Geometry: final body of the model. Coordinates: model frame, mm. A direction names the side the tool comes from. Give positions to 0.01 mm unless a question says otherwise; leave off trailing zeros. Write each loop counter-clockwise with the first axis right and the second up, starting at its lowest first coordinate (ties: lowest second). Pieces come first, ordered by that corner, then holes. Notation, with made-up numbers: (-9.5, 14) - (35.5, 14) arc R26 cw to (35.5, 51) - close; hole circle Ø6 at (-24, 28.25). An arc over 180 degrees is marked (long way). Return JSON: item names as keys, results as strings.
Autodesk Inventor part; units mm, degrees
ref_plane "YZ Plane" through (0, 0, 0) normal (1, 0, 0) x (0, 1, 0)
ref_plane "XZ Plane" through (0, 0, 0) normal (0, 1, 0) x (-1, 0, 0)
ref_plane "XY Plane" through (0, 0, 0) normal (0, 0, 1) x (1, 0, 0)
sketch "Sketch1" plane through (0, 0, 0) normal (0, 1, 0) x (-1, 0, 0)
  line L0 (0, 0) -> (-29.0466, 0)
  line L1 (0, 58.5031) -> (-5.7395, 64.2426)
  line L2 (6.2813, 43.0294) -> (-10.3357, 59.6464)
  line L3 (-10.3357, 59.6464) -> (-1.1433, 68.8388)
  line L4 (-1.1433, 68.8388) -> (15.4737, 52.2218)
  line L5 (15.4737, 52.2218) -> (6.2813, 43.0294)
  line L6 (6.2813, 43.0294) -> (-1.1433, 68.8388) construction
  line L7 (-10.3357, 59.6464) -> (15.4737, 52.2218) construction
  line L8 (7.802, 36.0648) -> (-17.3003, 61.1671)
  line L9 (-17.3003, 61.1671) -> (-2.664, 75.8034)
  line L10 (-2.664, 75.8034) -> (22.4383, 50.7011)
  line L11 (22.4383, 50.7011) -> (7.802, 36.0648)
  line L12 (7.802, 36.0648) -> (-2.664, 75.8034) construction
  line L13 (-17.3003, 61.1671) -> (22.4383, 50.7011) construction
  line L14 (7.802, 36.0648) -> (7.802, -0.7306)
  line L15 (22.4383, 50.7011) -> (22.4383, -0.4008)
  line L16 (6.2813, -43.0294) -> (-10.3357, -59.6464)
  line L17 (-10.3357, -59.6464) -> (-1.1433, -68.8388)
  line L18 (-1.1433, -68.8388) -> (15.4737, -52.2218)
  line L19 (15.4737, -52.2218) -> (6.2813, -43.0294)
  line L20 (-10.3357, -59.6464) -> (15.4737, -52.2218) construction
  line L21 (7.802, -36.0648) -> (-17.3003, -61.1671)
  line L22 (-17.3003, -61.1671) -> (-2.664, -75.8034)
  line L23 (-2.664, -75.8034) -> (22.4383, -50.7011)
  line L24 (22.4383, -50.7011) -> (7.802, -36.0648)
  line L25 (7.802, -36.0648) -> (-2.664, -75.8034) construction
  line L26 (7.802, -36.0648) -> (7.802, -0.7306)
  line L27 (22.4383, -50.7011) -> (22.4383, -0.4008)
  point P0 (2.569, 55.9341)
  point P1 (-1.4969, 60)
  dimension "d0" = 45
  dimension "d1" = 6
  dimension "d2" = 23.5
  dimension "d3" = 13
  dimension "d4" = 60
  dimension "d6" = 6
extrude "Extrusion1" add sketch "Sketch1" along normal blind 6
sketch "Sketch3" plane through (0, 0, 0) normal (0, -1, 0) x (1, 0, 0)
  line L0 (-9.3663, 0) -> (-22.4383, 0)
  line L1 (-22.4383, -50.7011) -> (-22.4383, 50.7011)
  circle A0 centre (-15.2967, -35) radius 3.75
  circle A1 centre (-15.2967, 0) radius 3.75
  circle A2 centre (-15.2967, -17.5) radius 3.75
  circle A3 centre (-15.2967, 35) radius 3.75
  line L2 (-19.0467, -35) -> (-17.1717, -31.7524)
  line L3 (-17.1717, -31.7524) -> (-13.4217, -31.7524)
  line L4 (-13.4217, -31.7524) -> (-11.5467, -35)
  line L5 (-11.5467, -35) -> (-13.4217, -38.2476)
  line L6 (-13.4217, -38.2476) -> (-17.1717, -38.2476)
  line L7 (-17.1717, -38.2476) -> (-19.0467, -35)
  line L8 (-19.0467, -17.5) -> (-17.1717, -14.2524)
  line L9 (-17.1717, -14.2524) -> (-13.4217, -14.2524)
  line L10 (-13.4217, -14.2524) -> (-11.5467, -17.5)
  line L11 (-11.5467, -17.5) -> (-13.4217, -20.7476)
  line L12 (-13.4217, -20.7476) -> (-17.1717, -20.7476)
  line L13 (-17.1717, -20.7476) -> (-19.0467, -17.5)
  line L14 (-19.0467, 0) -> (-17.1717, 3.2476)
  line L15 (-17.1717, 3.2476) -> (-13.4217, 3.2476)
  line L16 (-13.4217, 3.2476) -> (-11.5467, 0)
  line L17 (-11.5467, 0) -> (-13.4217, -3.2476)
  line L18 (-13.4217, -3.2476) -> (-17.1717, -3.2476)
  line L19 (-17.1717, -3.2476) -> (-19.0467, 0)
  line L20 (-19.0467, 35) -> (-17.1717, 38.2476)
  line L21 (-17.1717, 38.2476) -> (-13.4217, 38.2476)
  line L22 (-13.4217, 38.2476) -> (-11.5467, 35)
  line L23 (-11.5467, 35) -> (-13.4217, 31.7524)
  line L24 (-13.4217, 31.7524) -> (-17.1717, 31.7524)
  line L25 (-17.1717, 31.7524) -> (-19.0467, 35)
  circle A4 centre (-15.2967, 17.5) radius 3.75
  line L26 (-19.0467, 17.5) -> (-17.1717, 20.7476)
  line L27 (-17.1717, 20.7476) -> (-13.4217, 20.7476)
  line L28 (-13.4217, 20.7476) -> (-11.5467, 17.5)
  line L29 (-11.5467, 17.5) -> (-13.4217, 14.2524)
  line L30 (-13.4217, 14.2524) -> (-17.1717, 14.2524)
  line L31 (-17.1717, 14.2524) -> (-19.0467, 17.5)
  point P0 (0, 0)
  dimension "d15" = 7.5
  dimension "d16" = 7.5
  dimension "d17" = 7.5
  dimension "d19" = 7.5
  dimension "d20" = 7.5
extrude "Extrusion3" cut sketch "Sketch3" against normal blind 6 contours L17 L18 L19 L0 | L0 L14 L15 L16 | L5 L6 L7 L2 L3 L4 | L11 L12 L13 L8 L9 L10 | L23 L24 L25 L20 L21 L22 | L29 L30 L31 L26 L27 L28
sketch "Sketch5" plane through (0, 6, 0) normal (0, 1, 0) x (1, 0, 0)
  line L0 (-17.1717, -3.2476) -> (-19.0467, 0)
  line L1 (-19.0467, 0) -> (-17.1717, 3.2476)
  line L2 (-17.1717, 3.2476) -> (-13.4217, 3.2476)
  line L3 (-13.4217, 3.2476) -> (-11.5467, 0)
  line L4 (-11.5467, 0) -> (-13.4217, -3.2476)
  line L5 (-13.4217, -3.2476) -> (-17.1717, -3.2476)
  line L6 (-13.4217, 20.7476) -> (-11.5467, 17.5)
  line L7 (-11.5467, 17.5) -> (-13.4217, 14.2524)
  line L8 (-13.4217, 14.2524) -> (-17.1717, 14.2524)
  line L9 (-17.1717, 14.2524) -> (-19.0467, 17.5)
  line L10 (-19.0467, 17.5) -> (-17.1717, 20.7476)
  line L11 (-17.1717, 20.7476) -> (-13.4217, 20.7476)
  line L12 (-13.4217, -31.7524) -> (-11.5467, -35)
  line L13 (-11.5467, -35) -> (-13.4217, -38.2476)
  line L14 (-13.4217, -38.2476) -> (-17.1717, -38.2476)
  line L15 (-17.1717, -38.2476) -> (-19.0467, -35)
  line L16 (-19.0467, -35) -> (-17.1717, -31.7524)
  line L17 (-17.1717, -31.7524) -> (-13.4217, -31.7524)
  line L18 (-13.4217, 38.2476) -> (-11.5467, 35)
  line L19 (-11.5467, 35) -> (-13.4217, 31.7524)
  line L20 (-13.4217, 31.7524) -> (-17.1717, 31.7524)
  line L21 (-17.1717, 31.7524) -> (-19.0467, 35)
  line L22 (-19.0467, 35) -> (-17.1717, 38.2476)
  line L23 (-17.1717, 38.2476) -> (-13.4217, 38.2476)
  line L24 (-13.4217, -14.2524) -> (-11.5467, -17.5)
  line L25 (-11.5467, -17.5) -> (-13.4217, -20.7476)
  line L26 (-13.4217, -20.7476) -> (-17.1717, -20.7476)
  line L27 (-17.1717, -20.7476) -> (-19.0467, -17.5)
  line L28 (-19.0467, -17.5) -> (-17.1717, -14.2524)
  line L29 (-17.1717, -14.2524) -> (-13.4217, -14.2524)
  line L30 (-7.802, -36.0648) -> (-7.802, 36.0648)
  line L31 (-7.802, 36.0648) -> (17.3003, 61.1671)
  line L32 (17.3003, 61.1671) -> (2.664, 75.8034)
  line L33 (2.664, 75.8034) -> (-22.4383, 50.7011)
  line L34 (-22.4383, 50.7011) -> (-22.4383, -50.7011)
  line L35 (-22.4383, -50.7011) -> (2.664, -75.8034)
  line L36 (2.664, -75.8034) -> (17.3003, -61.1671)
  line L37 (17.3003, -61.1671) -> (-7.802, -36.0648)
  line L38 (1.1433, 68.8388) -> (10.3357, 59.6464)
  line L39 (10.3357, 59.6464) -> (-6.2813, 43.0294)
  line L40 (-6.2813, 43.0294) -> (-15.4737, 52.2218)
  line L41 (-15.4737, 52.2218) -> (1.1433, 68.8388)
  line L42 (1.1433, -68.8388) -> (-15.4737, -52.2218)
  line L43 (-15.4737, -52.2218) -> (-6.2813, -43.0294)
  line L44 (-6.2813, -43.0294) -> (10.3357, -59.6464)
  line L45 (10.3357, -59.6464) -> (1.1433, -68.8388)
  line L46 (-13.4217, -31.7524) -> (-11.5467, -35)
  line L47 (-11.5467, -35) -> (-7.802, -35)
  line L48 (-7.802, -36.0648) -> (-7.802, 36.0648)
  line L49 (-11.5467, -17.5) -> (-7.802, -17.5)
  line L50 (-11.5467, 17.5) -> (-7.802, 17.5)
  line L51 (-13.4217, 31.7524) -> (-11.5467, 35)
  line L52 (-11.5467, 35) -> (-7.802, 35)
  line L53 (-7.802, -26.25) -> (-16.5311, -26.25)
  line L54 (-7.802, 26.25) -> (-17.8697, 26.25)
  circle A0 centre (-13.302, -26.25) radius 2.05
  circle A1 centre (-13.302, 26.25) radius 2.05
  point P0 (0, 0)
  dimension "d34" = 8.75
  dimension "d35" = 8.75
  dimension "d38" = 4.1
  dimension "d39" = 5.5
  dimension "d40" = 4.1
  dimension "d41" = 5.5
extrude "Extrusion4" cut sketch "Sketch5" against normal blind 10 contours A1 L54 | L54 A1 | A0 L53 | L53 A0
chamfer "Chamfer1" distance 1 angle 45 8 edges at (-7.802, 6, 0) (-22.4383, 6, 0) (4.7492, 6, 48.616) (9.9822, 6, 68.4853) (-9.8871, 6, 63.2523) (4.7492, 6, -48.616) (-9.8871, 6, -63.2523) (9.9822, 6, -68.4853)
chamfer "Chamfer2" distance 0.5 angle 45 30 edges at (-15.2967, 6, 3.2476) (-18.1092, 6, 1.6238) (-18.1092, 6, -1.6238) (-15.2967, 6, -3.2476) (-12.4842, 6, -1.6238) (-12.4842, 6, 1.6238) (-15.2967, 6, -14.2524) (-18.1092, 6, -15.8762) (-18.1092, 6, -19.1238) (-15.2967, 6, -20.7476) (-12.4842, 6, -19.1238) (-12.4842, 6, -15.8762) (-18.1092, 6, -33.3762) (-18.1092, 6, -36.6238) (-15.2967, 6, -38.2476) (-12.4842, 6, -36.6238) (-12.4842, 6, -33.3762) (-15.2967, 6, -31.7524) (-15.2967, 6, 14.2524) (-18.1092, 6, 15.8762) (-18.1092, 6, 19.1238) (-15.2967, 6, 20.7476) (-12.4842, 6, 19.1238) (-12.4842, 6, 15.8762) (-15.2967, 6, 31.7524) (-18.1092, 6, 33.3762) (-18.1092, 6, 36.6238) (-15.2967, 6, 38.2476) (-12.4842, 6, 36.6238) (-12.4842, 6, 33.3762)
sketch "Sketch6" plane through (0, 6, 0) normal (0, 1, 0) x (1, 0, 0)
  circle A0 centre (-13.302, -26.25) radius 2.05
  circle A1 centre (-13.302, -26.25) radius 3.5
  circle A2 centre (-13.302, 26.25) radius 2.05
  circle A3 centre (-13.302, 26.25) radius 3.5
  point P0 (0, 0)
  dimension "d50" = 7
  dimension "d51" = 7
extrude "Extrusion5" cut sketch "Sketch6" against normal blind 3
equation "\"d15\" = d17"
equation "\"d16\" = d17"
equation "\"d19\" = d17"
equation "\"d20\" = d17"
equation "\"d51\" = d50"
properties part number "Side_Frame"
Q1. Mould query, pull axis X, two halves, no side actions, for faces 1 (the flat face through (-11, 3, 26)), 2 (the flat face through (-9.71, 2.46, 63.43)), 3 (the flat face through (1.91, 2.96, 51.22)). Classes: pulls with the +X half, pulls with the -X half, needs draft (parallel to the pull), parting line crosses it, or undercut.
Answer key:
{"face 1": "undercut", "face 2": "pulls with the -X half", "face 3": "undercut"}
Q2. Section query C-C, the plane z = -9. Return the cut outline in (x, y).
Answer key:
{"outline": "(-22.44, 0) - (-7.8, 0) - (-7.8, 5) - (-8.8, 6) - (-21.44, 6) - (-22.44, 5) - close"}
Q3. Section query B-B, the plane x = 4. Return the cut outline in (y, z), plus the area to 3 significant figures.
Answer key:
{"outline": "(0, -74.47) - (5, -74.47) - (6, -73.05) - (6, -65.98) - (0, -65.98) - close; (0, -53.31) - (6, -53.31) - (6, -49.28) - (5, -47.87) - (0, -47.87) - close; (0, 47.87) - (5, 47.87) - (6, 49.28) - (6, 53.31) - (0, 53.31) - close; (0, 65.98) - (6, 65.98) - (6, 73.05) - (5, 74.47) - (0, 74.47) - close", "area": "164 mm^2"}
Q4. Pin query (flat end, axial travel): P1, Ø3, axis at x = -16, y = 2.5, coming from the -Z side; P2, Ø3, axis at x = -15.5, y = 2.5, coming from the -Z side; P3, Ø3, axis at x = -15, y = 3, coming from the +Z side. Return the tip coordinate at first contact, or that it passes through.
Answer key:
{"P1": "stops at z = -58.64", "P2": "stops at z = -59.14", "P3": "stops at z = 59.64"}
Q5. Material intervals for probe 1 along X at (y, z) = (4.75, 26.25); probe 2 along Z at (x, y) = (-18.5, 3.25); probe 3 along Z at (x, y) = (8, 4.5), sorted ascending. Write a range as [from, to].
Answer key:
{"probe 1": "x = [-22.44, -16.8], [-9.8, -7.8]", "probe 2": "z = [-54.64, -35.95], [-34.05, -18.45], [-16.55, -0.95], [0.95, 16.55], [18.45, 34.05], [35.95, 54.64]", "probe 3": "z = [-70.47, -61.98], [-57.31, -51.87], [51.87, 57.31], [61.98, 70.47]"}
Q6. Section query A-A, the plane z = 26.25. Return the cut outline in (x, y).
Answer key:
{"outline": "(-22.44, 0) - (-15.35, 0) - (-15.35, 3) - (-16.8, 3) - (-16.8, 6) - (-21.44, 6) - (-22.44, 5) - close; (-11.25, 0) - (-7.8, 0) - (-7.8, 5) - (-8.8, 6) - (-9.8, 6) - (-9.8, 3) - (-11.25, 3) - close"}
Q7. Section query D-D, the plane z = 49. Return the cut outline in (x, y).
Answer key:
{"outline": "(-22.44, 0) - (-12.25, 0) - (-12.25, 6) - (-21.44, 6) - (-22.44, 5) - close; (-0.31, 0) - (5.13, 0) - (5.13, 5) - (3.72, 6) - (-0.31, 6) - close"}
Q8. Set-up query: faces 4 (the flat face through (-18.34, 5.75, -15.78)), 5 (the flat face through (-15, 3, 20.748)). Return all of +Z, -Z, +X, -X, +Y, -Y with unobstructed straight access to the full face (end or side cutting, diameter ignored); none if empty.
Answer key:
{"face 4": "+Y", "face 5": "+Y, -Y"}
